Design review of the part built by this model. Coordinates are the model's own, in mm. Face numbers are marked on the shaded views. A direction names the side the tool comes from. Round coordinates to 2 decimals unless told otherwise and drop trailing zeros. Loops run counter-clockwise (first coordinate to the right, second up) from the corner with the lowest first, then second, coordinate; pieces in that order, holes last. Notation, with made-up numbers: (19, 64.25) - (56, 64.25) arc R17 cw to (56, 87.25) - close; hole circle Ø5 at (-25, 9.5). An arc over 180 degrees is marked (long way). Return JSON: item names as keys, results as strings. Group by question number.
(1) We need section D-D, the plane x = -32.75. Write out the cut boundary in (y, z).
(2) We need section B-B, the plane y = 1.2. Write out the cut boundary in (x, z), and give its area (3 significant figures).
(3) We need section C-C, the plane z = -6.75. Write out the cut boundary in (x, y), and give its area (3 significant figures).
(4) The part is to be moulded in two halves that separate along X. For the marked faces 3, 4 and 5, say which applies: pulls with the +X half, pulls with the -X half, needs draft (parallel to the pull), parting line crosses it, or undercut.
(5) Clearance check with flat-ended pins moving along their axes: pin 1 (0.5 mm diameter, centred on x = -34.5, y = 1, fed in from -Z); pin 2 (0.9 mm diameter, centred on x = -29, y = 1.5, fed in from +Z); pin 3 (1 mm diameter, centred on y = 2, z = -3.5, fed in from +X). State where each tip first meets the part, or that it passes through.
(6) For the marked faces 1 and 2, list the 3-axis set-ups (+Z, -Z, +X, -X, +Y, -Y) from which the entire face can be reached by the end or side of a thin tool; tool diameter is ignored.
(7) Wall thickness on L1, parallel to X at y = 1.15, z = 4.5; L2, parallel to Z at x = -30, y = 2.3; L3, parallel to X at y = 2.6, z = -2.5: over which ranges is each line inside the solid? List them lowest first. Write a range as [from, to].
(8) We need section A-A, the plane z = 3.25. Write out the cut boundary in (x, y).
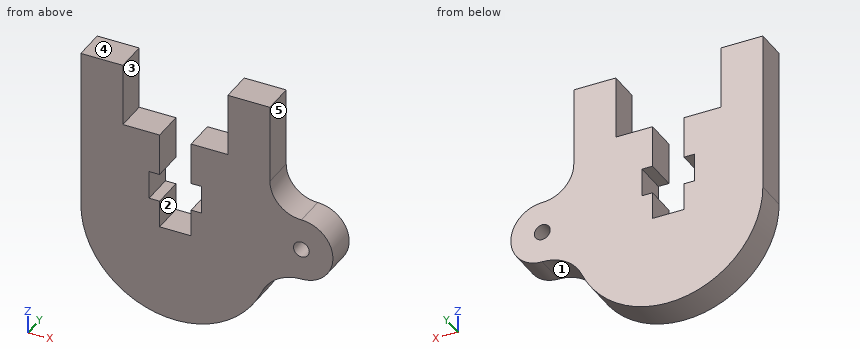
from build123d import *

# Parameters (mm, degrees)
SKETCH_1_R      = 0.75
EXTRUDE_1_DEPTH = 3


with BuildPart() as part:
    # 草图1 → 凸台-拉伸1 (new body)
    with BuildSketch(Plane(origin=(0, 0, 0), x_dir=(1, 0, 0), z_dir=(0, 1, 0))):
        with BuildLine():
            Line((-41.303773208, 8.184389917), (-41.303773208, -7.115610083))
            Line((-41.303773208, -7.115610083), (-37.303773208, -7.115610083))
            Line((-37.303773208, -7.115610083), (-37.303773208, -1.115610083))
            Line((-37.303773208, -1.115610083), (-33.803773208, -1.115610083))
            Line((-33.803773208, -1.115610083), (-33.803773208, 2.884389917))
            Line((-33.803773208, 2.884389917), (-34.803773208, 2.884389917))
            Line((-34.803773208, 2.884389917), (-34.803773208, 5.584389917))
            Line((-34.803773208, 5.584389917), (-33.803773208, 5.584389917))
            Line((-33.803773208, 5.584389917), (-33.803773208, 8.184389917))
            Line((-33.803773208, 8.184389917), (-30.803773208, 8.184389917))
            Line((-30.803773208, 8.184389917), (-30.803773208, 5.584389917))
            Line((-30.803773208, 5.584389917), (-29.803773208, 5.584389917))
            Line((-29.803773208, 5.584389917), (-29.803773208, 2.884389917))
            Line((-29.803773208, 2.884389917), (-30.803773208, 2.884389917))
            Line((-30.803773208, 2.884389917), (-30.803773208, -1.115610083))
            Line((-30.803773208, -1.115610083), (-27.303773208, -1.115610083))
            Line((-27.303773208, -1.115610083), (-27.303773208, -7.115610083))
            Line((-27.303773208, -7.115610083), (-23.303773208, -7.115610083))
            Line((-23.303773208, -7.115610083), (-23.303773208, 0.384389917))
            ThreePointArc((-23.303773208, 0.384389917), (-22.425093551, 2.505710261), (-20.303773208, 3.384389917))
            ThreePointArc((-20.303773208, 3.384389917), (-17.303773208, 6.384389917), (-20.303773208, 9.384389917))
            ThreePointArc((-20.303773208, 9.384389917), (-22.554994318, 10.051742056), (-24.078817144, 11.838168476))
            ThreePointArc((-24.078817144, 11.838168476), (-34.171311083, 16.988497043), (-41.303773208, 8.184389917))
        make_face()
        with Locations(Location((-20.303773208, 6.384389917, 0), (0, 0, 270))):
            Circle(SKETCH_1_R, mode=Mode.SUBTRACT)
    extrude(amount=EXTRUDE_1_DEPTH)


solid = part.part
Solutions:
{
 "1": {"outline": "(0, -17.17) - (3, -17.17) - (3, -8.18) - (0, -8.18) - close"},
 "2": {"outline": "(-41.3, -8.18) arc R9 ccw to (-24.08, -11.84) arc R4.13 cw to (-20.3, -9.38) arc R3 ccw to (-20.3, -3.38) arc R3 cw to (-23.3, -0.38) - (-23.3, 7.12) - (-27.3, 7.12) - (-27.3, 1.12) - (-30.8, 1.12) - (-30.8, -2.88) - (-29.8, -2.88) - (-29.8, -5.58) - (-30.8, -5.58) - (-30.8, -8.18) - (-33.8, -8.18) - (-33.8, -5.58) - (-34.8, -5.58) - (-34.8, -2.88) - (-33.8, -2.88) - (-33.8, 1.12) - (-37.3, 1.12) - (-37.3, 7.12) - (-41.3, 7.12) - close; hole circle Ø1.5 at (-20.3, -6.38)", "area": "343 mm^2"},
 "3": {"outline": "(-41.3, 0) - (-33.8, 0) - (-33.8, 3) - (-41.3, 3) - close; (-30.8, 0) - (-20.96, 0) - (-20.96, 3) - (-30.8, 3) - close; (-19.65, 0) - (-17.33, 0) - (-17.33, 3) - (-19.65, 3) - close", "area": "59.0 mm^2"},
 "4": {"face 3": "undercut", "face 4": "needs draft", "face 5": "pulls with the +X half"},
 "5": {"pin 1": "z = -16.97", "pin 2": "z = 1.12", "pin 3": "x = -18.48"},
 "6": {"face 1": "-Z, +X, +Y, -Y", "face 2": "+Z, +Y, -Y"},
 "7": {"L1": "[-41.3, -37.3], [-27.3, -23.3]", "L2": "[-16.88, -5.58], [-2.88, 1.12]", "L3": "[-41.3, -33.8], [-30.8, -22.43]"},
 "8": {"outline": "(-41.3, 0) - (-37.3, 0) - (-37.3, 3) - (-41.3, 3) - close; (-27.3, 0) - (-23.3, 0) - (-23.3, 3) - (-27.3, 3) - close"}
}
